Can you work these out from the drawing? Everything is in mm from the part's minimum corner. A direction names the side the tool comes from. Give positions to 0.01 mm unless a question says otherwise; leave off trailing zeros. Write each loop counter-clockwise with the first axis right and the second up, starting at its lowest first coordinate (ties: lowest second). Pieces come first, ordered by that corner, then holes. Notation, with made-up numbers: (-1, 7) - (40, 7) arc R20 ccw to (40, 46) - close; hole circle Ø3 at (22.5, 26). An arc over 180 degrees is marked (long way). Write each question's results on one line, items separated by ' | '. Start each with the question number.
Item 1: We'd pull the mould along X, two halves only. Please class the marked faces 3, 4 and 5: +X half, -X half, draft (parallel to the pull), parting line (faces both ways), or undercut.
Item 2: Suppose I cut it at C-C on y = 3. List the corners of the cut face in (x, z) for me.
Item 3: Will these pins go through, and if not, where does the flat tip stop? P1, Ø19, axis at x = 17.5, z = 17.5, coming from the -Y side; P2, Ø1.5, axis at x = 29, y = 2, coming from the -Z side; P3, Ø1, axis at y = 6, z = 20.5, coming from the +X side; P4, Ø4.5, axis at x = 17.5, z = 17.5, coming from the -Y side.
Item 4: Which directions (+Z, -Z, +X, -X, +Y, -Y) give clear straight access to the entire face, cutting with the end or side of a thin tool? Please do the marked faces 1 and 2.
Item 5: Suppose I cut it at D-D on x = 7.5. List the corners of the cut face in (y, z) for me, then the cut area to 3 significant figures.
Item 6: Suppose I cut it at A-A on x = 17.5. List the corners of the cut face in (y, z) for me.
Item 7: Please list where these lines run through material, in increasing order: line 1 along Z through (x, y) = (17.5, 2.25); line 2 along Z through (x, y) = (18.5, 1.75); line 3 along Y through (x, z) = (8, 24.5).
Item 8: Suppose I cut it at B-B on z = 17.5. List the corners of the cut face in (x, y) for me, then the cut area to 3 significant figures.
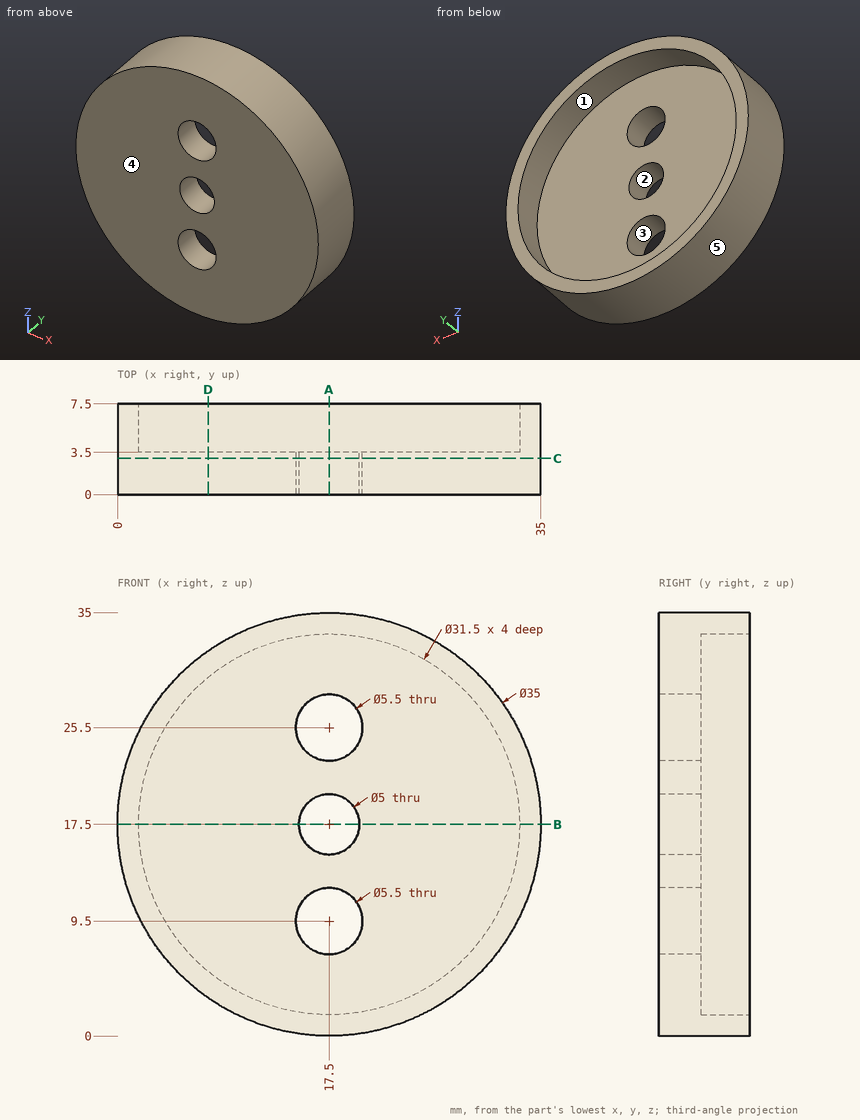
Checked values:
1) face 3: undercut | face 4: draft | face 5: parting line
2) outline: circle Ø35 at (17.5, 17.5); hole circle Ø5.5 at (17.5, 9.5); hole circle Ø5.5 at (17.5, 25.5); hole circle Ø5 at (17.5, 17.5)
3) P1: stops at y = 0 | P2: stops at z = 3.69 | P3: stops at x = 34.82 | P4: passes through
4) face 1: +Y | face 2: +Y, -Y
5) outline: (0, 3.14) - (7.5, 3.14) - (7.5, 5.33) - (3.5, 5.33) - (3.5, 29.67) - (7.5, 29.67) - (7.5, 31.86) - (0, 31.86) - close | area: 118 mm^2
6) outline: (0, 0) - (7.5, 0) - (7.5, 1.75) - (3.5, 1.75) - (3.5, 6.75) - (0, 6.75) - close; (0, 12.25) - (3.5, 12.25) - (3.5, 15) - (0, 15) - close; (0, 20) - (3.5, 20) - (3.5, 22.75) - (0, 22.75) - close; (0, 28.25) - (3.5, 28.25) - (3.5, 33.25) - (7.5, 33.25) - (7.5, 35) - (0, 35) - close
7) line 1: z = 0 to 6.75, 12.25 to 15, 20 to 22.75, 28.25 to 35 | line 2: z = 0.03 to 6.94, 12.06 to 15.21, 19.79 to 22.94, 28.06 to 34.97 | line 3: y = 0 to 3.5
8) outline: (0, 0) - (15, 0) - (15, 3.5) - (1.75, 3.5) - (1.75, 7.5) - (0, 7.5) - close; (20, 0) - (35, 0) - (35, 7.5) - (33.25, 7.5) - (33.25, 3.5) - (20, 3.5) - close | area: 119 mm^2
